Autodesk Inventor part; units mm, degrees
ref_plane "Work Plane1" through (-250, -12.35, -20) normal (0, 0, -1) x (0, 1, 0)
ref_plane "YZ Plane" through (0, 0, 0) normal (1, 0, 0) x (0, 1, 0)
ref_plane "XZ Plane" through (0, 0, 0) normal (0, 1, 0) x (-1, 0, 0)
sketch "Sketch1" plane through (0, 0, 0) normal (0, 0, 1) x (1, 0, 0)
  circle A0 centre (-131.3, 44.85) radius 1.5
  circle A1 centre (-147.3, 44.85) radius 1.5
  circle A2 centre (-139.3, 52.85) radius 1.5
  circle A3 centre (-139.3, 36.85) radius 1.5
  circle A4 centre (-139.3, 44.85) radius 4
  circle A5 centre (-139.3, 44.85) radius 11
  line L0 (-250, 102.05) -> (-125, 102.05)
  line L1 (-250, 96.9) -> (-250, 102.05)
  line L2 (-125, 96.9) -> (-250, 96.9)
  line L3 (-125, 96.9) -> (-125, 102.05)
  line L4 (-125, 103.3) -> (-250, 103.3)
  line L5 (-125, 84.55) -> (-250, 84.55)
  line L6 (-125, 84.55) -> (-125, 89.7)
  line L7 (-125, 89.7) -> (-250, 89.7)
  line L8 (-250, 84.55) -> (-250, 89.7)
  line L9 (-250, 83.3) -> (-125, 83.3)
  line L10 (-250, 5.15) -> (-125, 5.15)
  line L11 (-250, 0) -> (-250, 5.15)
  line L12 (0, 0) -> (-250, 0)
  line L13 (-125, 0) -> (-125, 5.15)
  line L14 (-125, -12.35) -> (-250, -12.35)
  line L15 (-125, -12.35) -> (-125, -7.2)
  line L16 (-125, -7.2) -> (-250, -7.2)
  line L17 (-250, -12.35) -> (-250, -7.2)
  line L18 (-250, -13.6) -> (-125, -13.6)
  line L19 (-125, 6.4) -> (-250, 6.4)
  line L20 (-128.3, 103.3) -> (-150.3, 103.3)
  line L21 (-150.3, 103.3) -> (-150.3, -13.6)
  line L22 (-150.3, -13.6) -> (-128.3, -13.6)
  line L23 (-128.3, -13.6) -> (-128.3, 103.3)
  circle A6 centre (-139.3, 44.85) radius 5.5902
extrude "Extrusion1" add sketch "Sketch1" along normal blind 6.35 contours A5 | L23 L19 L21 A5 | A5 L21 L9 L23 | L23 L10 L21 L19 | L9 L21 L5 L23 | L23 L12 L21 L10 | L5 L21 L7 L23 | L23 L16 L21 L12 | L7 L21 L2 L23 | L23 L14 L21 L16 | L2 L21 L0 L23 | L23 L18 L21 L14 | L0 L21 L4 L23
sketch "Sketch2" plane through (0, 0, 0) normal (0, 0, -1) x (-1, 0, 0)
  line L0 (125, 5.15) -> (250, 5.15)
  line L1 (125, 5.15) -> (125, 0)
  line L2 (125, 0) -> (250, 0)
  line L3 (250, 5.15) -> (250, 0)
  line L4 (250, 6.4) -> (125, 6.4)
  line L5 (250, 84.55) -> (125, 84.55)
  line L6 (250, 89.7) -> (250, 84.55)
  line L7 (125, 89.7) -> (250, 89.7)
  line L8 (125, 89.7) -> (125, 84.55)
  line L9 (125, 83.3) -> (250, 83.3)
  circle A0 centre (139.3, 44.85) radius 5.5902
  circle A1 centre (139.3, 36.85) radius 1.5
  circle A2 centre (139.3, 52.85) radius 1.5
  circle A3 centre (147.3, 44.85) radius 1.5
  circle A4 centre (131.3, 44.85) radius 1.5
  line L10 (128.3, 103.3) -> (150.3, 103.3)
  line L11 (128.3, -13.6) -> (128.3, 103.3)
  line L12 (150.3, -13.6) -> (128.3, -13.6)
  line L13 (150.3, 103.3) -> (150.3, -13.6)
  line L14 (128.3, -13.6) -> (128.3, 103.3)
  line L15 (150.3, 103.3) -> (150.3, -13.6)
  line L16 (128.3, 6.4) -> (150.3, 6.4)
  line L17 (150.3, 6.4) -> (150.3, 12.75)
  line L18 (150.3, 12.75) -> (128.3, 12.75)
  line L19 (128.3, 12.75) -> (128.3, 6.4)
  line L20 (128.3, 83.3) -> (150.3, 83.3)
  line L21 (150.3, 83.3) -> (150.3, 76.95)
  line L22 (150.3, 76.95) -> (128.3, 76.95)
  line L23 (128.3, 76.95) -> (128.3, 83.3)
  point P0 (0, 0)
  dimension "d2" = 6.35
  dimension "d3" = 6.35
ref_plane "Work Plane1" through (-250, -12.35, -20) normal (0, 0, -1) x (0, 1, 0)
extrude "Extrusion2" add sketch "Sketch2" along normal up to surface (20 mm away) contours L11 L18 L13 L4 | L11 L9 L13 L22
sketch "Sketch3" plane through (-128.3, -13.6, 6.35) normal (1, 0, 0) x (0, 0, -1)
  line L0 (6.35, 26.35) -> (26.35, 26.35)
  line L1 (26.35, 26.35) -> (6.35, 46.35)
  line L2 (6.35, 26.35) -> (6.35, 90.55)
  line L3 (6.35, 90.55) -> (26.35, 90.55)
  line L4 (26.35, 90.55) -> (6.35, 70.55)
  line L5 (6.35, 70.55) -> (6.35, 90.55)
  line L6 (26.35, 90.55) -> (6.35, 90.55)
  line L7 (6.35, 46.35) -> (6.35, 26.35)
  line L8 (26.35, 26.35) -> (6.35, 26.35)
  point P0 (6.35, 13.6)
  dimension "d6" = 45
  dimension "d7" = 45
extrude "Extrusion3" add sketch "Sketch3" against normal up to surface (22 mm away)
sketch "Sketch4" plane through (-128.3, 83.3, -20) normal (0, 0, -1) x (-1, 0, 0)
  line L0 (0, 0) -> (22, 0)
  line L1 (0, -6.35) -> (0, 0)
  line L2 (22, -6.35) -> (0, -6.35)
  line L3 (22, 0) -> (22, -6.35)
  line L4 (0, -76.9) -> (0, -70.55)
  line L5 (22, -76.9) -> (0, -76.9)
  line L6 (22, -70.55) -> (22, -76.9)
  line L7 (0, -70.55) -> (22, -70.55)
  line L8 (22, -26.35) -> (22, -6.35)
  line L9 (22, -6.35) -> (0, -6.35)
  line L10 (0, -26.35) -> (0, -6.35)
  line L11 (22, -26.35) -> (0, -26.35)
  line L12 (22, -70.55) -> (22, -50.55)
  line L13 (0, -50.55) -> (22, -50.55)
  line L14 (0, -70.55) -> (0, -50.55)
  line L15 (0, -70.55) -> (22, -70.55)
  line L16 (22, -6.35) -> (0, -6.35)
  line L17 (11, -6.35) -> (11, -70.55)
  line L18 (0, -70.55) -> (22, -70.55)
  line L19 (19.46, -70.55) -> (2.54, -70.55)
  line L20 (2.54, -70.55) -> (2.54, -6.35)
  line L21 (2.54, -6.35) -> (19.46, -6.35)
  line L22 (19.46, -6.35) -> (19.46, -70.55)
  line L23 (19.46, -70.55) -> (2.54, -6.35) construction
  line L24 (2.54, -70.55) -> (19.46, -6.35) construction
  point P0 (-128.3, -83.3)
  point P1 (11, -38.45)
  dimension "d10" = 2.54
extrude "Extrusion4" cut sketch "Sketch4" against normal up to surface (20 mm away) contours L2 L17 L11 L20 | L22 L11 L17 L2 | L11 L17 L13 L20 | L22 L13 L17 L11 | L13 L17 L7 L20 | L22 L7 L17 L13
sketch "Sketch5" plane through (-150.3, 6.4, 0) normal (0, -1, 0) x (1, 0, 0)
  line L0 (0, -20) -> (22, -20)
  line L1 (2.54, 0) -> (0, 0)
  line L2 (22, -20) -> (0, 0)
  circle A0 centre (11, -10) radius 2.75
  point P0 (150.3, 0)
  dimension "d13" = 5.5
extrude "Extrusion5" cut sketch "Sketch5" against normal through all
sketch "Sketch6" plane through (0, 0, 0) normal (0, 0, -1) x (-1, 0, 0)
  line L0 (128.3, 83.3) -> (150.3, 83.3)
  line L1 (128.3, 76.95) -> (128.3, 83.3)
  line L2 (130.84, 76.95) -> (128.3, 76.95)
  line L3 (147.76, 76.95) -> (130.84, 76.95)
  line L4 (150.3, 76.95) -> (147.76, 76.95)
  line L5 (150.3, 83.3) -> (150.3, 76.95)
  line L6 (128.3, 6.4) -> (128.3, 12.75)
  line L7 (150.3, 6.4) -> (128.3, 6.4)
  line L8 (150.3, 12.75) -> (150.3, 6.4)
  line L9 (147.76, 12.75) -> (150.3, 12.75)
  line L10 (130.84, 12.75) -> (147.76, 12.75)
  line L11 (128.3, 12.75) -> (130.84, 12.75)
  line L12 (128.3, 103.3) -> (150.3, 103.3)
  line L13 (150.3, -13.6) -> (128.3, -13.6)
  line L14 (139.3, 103.3) -> (139.3, 83.3)
  line L15 (139.3, 6.4) -> (139.3, -13.6)
  circle A0 centre (139.3, 93.3) radius 2.75
  circle A1 centre (139.3, -3.6) radius 2.75
  point P0 (0, 0)
  dimension "d16" = 5.5
extrude "Extrusion6" cut sketch "Sketch6" against normal through all contours A0 L14 | L14 A0 | A1 L15 | L15 A1
properties part number "ZNutHolder"
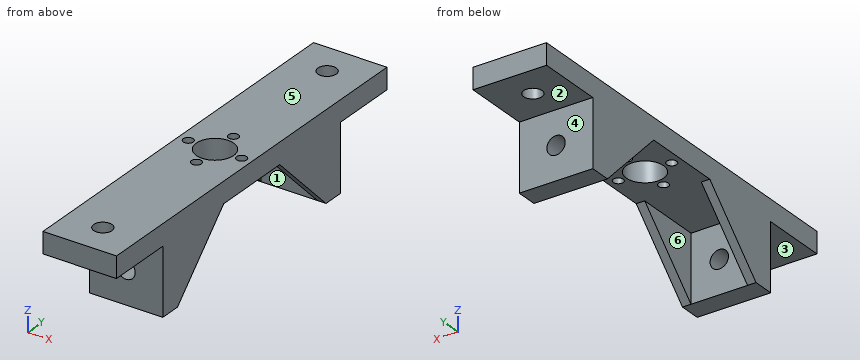
Read the model definition and answer for the solid it produces. Units are mm, in the model's axes. Face numbers are marked on the shaded views. A direction names the side the tool comes from. Round coordinates to 2 decimals unless told otherwise and drop trailing zeros. Order: outer loops, then holes, each group sorted by start corner. A loop starts at its lowest first (then second) coordinate and runs counter-clockwise, first axis right, second up.
1) Flat-ended cylindrical pins translate along their axes: pin 1 (6.5 mm diameter, centred on x = -139.3, y = 93.3, fed in from -Z); pin 2 (6 mm diameter, centred on x = -135.5, z = -10.5, fed in from +Y); pin 3 (10 mm diameter, centred on x = -140, z = -14.5, fed in from -Y). Find the tip coordinate at first contact, or state that the pin passes through.
2) Straight lines are drawn through the part: L1, parallel to X at y = 93.3, z = 2; L2, parallel to Y at x = -147.3, z = 5.25; L3, parallel to Y at x = -132.5, z = -10.75. For each, find the intervals that lie inside material, in ascending order.
3) The part is cut by section D-D on y = 44.85. Write down the section's boundary in (x, z), plus the area to 3 significant figures.
4) The part is cut by section C-C on z = -10. Write down the section's boundary in (x, y), plus the area to 3 significant figures.
5) The mould has two halves that part along Y. Classify the marked faces 4, 5 and 6: released by +Y, released by -Y, zero draft, split by the parting line, or undercut.
6) The part is cut by section A-A on z = -16.5. Write down the section's boundary in (x, y), plus the area to 3 significant figures.
7) The part is cut by section B-B on y = -3.6. Write down the section's boundary in (x, z).
8) For the marked faces 1, 2 and 3, determine the directions among +Z, -Z, +X, -X, +Y, -Y from which every point of the face is accessible in a straight line to the end or side of a thin tool.
Resolved:
1. pin 1: stops at z = 0
1. pin 2: stops at y = 83.3
1. pin 3: stops at y = 6.4
2. L1: x = -150.3 to -142.05, -136.55 to -128.3
2. L2: y = -13.6 to 43.35, 46.35 to 103.3
2. L3: y = 6.4 to 12.75, 76.95 to 83.3
3. outline: (-150.3, 0) - (-148.8, 0) - (-148.8, 6.35) - (-150.3, 6.35) - close; (-145.8, 0) - (-144.89, 0) - (-144.89, 6.35) - (-145.8, 6.35) - close; (-133.71, 0) - (-132.8, 0) - (-132.8, 6.35) - (-133.71, 6.35) - close; (-129.8, 0) - (-128.3, 0) - (-128.3, 6.35) - (-129.8, 6.35) - close
3. area: 30.6 mm2
4. outline: (-150.3, 6.4) - (-142.05, 6.4) - (-142.05, 12.75) - (-147.76, 12.75) - (-147.76, 22.75) - (-150.3, 22.75) - close; (-150.3, 66.95) - (-147.76, 66.95) - (-147.76, 76.95) - (-142.05, 76.95) - (-142.05, 83.3) - (-150.3, 83.3) - close; (-136.55, 6.4) - (-128.3, 6.4) - (-128.3, 22.75) - (-130.84, 22.75) - (-130.84, 12.75) - (-136.55, 12.75) - close; (-136.55, 76.95) - (-130.84, 76.95) - (-130.84, 66.95) - (-128.3, 66.95) - (-128.3, 83.3) - (-136.55, 83.3) - close
4. area: 311 mm2
5. face 4: released by +Y
5. face 5: zero draft
5. face 6: undercut
6. outline: (-150.3, 6.4) - (-128.3, 6.4) - (-128.3, 16.25) - (-130.84, 16.25) - (-130.84, 12.75) - (-147.76, 12.75) - (-147.76, 16.25) - (-150.3, 16.25) - close; (-150.3, 73.45) - (-147.76, 73.45) - (-147.76, 76.95) - (-130.84, 76.95) - (-130.84, 73.45) - (-128.3, 73.45) - (-128.3, 83.3) - (-150.3, 83.3) - close
6. area: 315 mm2
7. outline: (-150.3, 0) - (-142.05, 0) - (-142.05, 6.35) - (-150.3, 6.35) - close; (-136.55, 0) - (-128.3, 0) - (-128.3, 6.35) - (-136.55, 6.35) - close
8. face 1: -Z
8. face 2: -Z, +X, -X, +Y
8. face 3: -Z, +X, -X, -Y
